```python
from build123d import *

# Parameters (mm, degrees)
F0_R     = 10
F1_DEPTH = 2


with BuildPart() as f1:
    # F0 (on Front) → F1 (new body)
    with BuildSketch(Plane.XZ):
        with BuildLine():
            ThreePointArc((-62.534281, -2.119643), (-35.69599, 2.957285), (-15.866047, -15.826814))
            Line((-15.866047, -15.826814), (10.849682, -15.826814))
            Line((10.849682, -15.826814), (10.849682, 24.173186))
            ThreePointArc((10.849682, 24.173186), (-10.750328, 10.703225), (-13.3423, 36.026771))
            Line((-13.3423, 36.026771), (-62.534281, -2.119643))
        make_face()
        with BuildLine():
            ThreePointArc((10.849682, 24.173186), (2.449692, 37.643148), (-13.3423, 36.026771))
            ThreePointArc((-13.3423, 36.026771), (-10.750328, 10.703225), (10.849682, 24.173186))
        make_face()
        with Locations((-4.150318, 24.173186)):
            Circle(F0_R, mode=Mode.SUBTRACT)
        with BuildLine():
            Line((-44.150318, -15.826814), (-15.866047, -15.826814))
            ThreePointArc((-15.866047, -15.826814), (-35.69599, 2.957285), (-62.534281, -2.119643))
            ThreePointArc((-62.534281, -2.119643), (-61.408556, -50.365624), (-15.62346, -35.1122))
            Line((-15.62346, -35.1122), (-43.898783, -35.82365))
            ThreePointArc((-43.898783, -35.82365), (-54.149527, -25.952591), (-44.150318, -15.826814))
        make_face()
    extrude(amount=F1_DEPTH)


solid = f1.part
```
Geometry check sheet. Reference: the model listing, model coordinates, mm. Give positions to 0.01 mm unless a question says otherwise; leave off trailing zeros. Order: outer loops, then holes, each group sorted by start corner. A loop starts at its lowest first (then second) coordinate and runs counter-clockwise, first axis right, second up. Notation, with made-up numbers: (83, 29.5) - (100, 29.5) arc R21 ccw to (100, 62.5) - close; hole circle Ø4 at (-22, 26). An arc over 180 degrees is marked (long way). Answer in a Markdown table with one row per item. Add a question column.
Q1. Material ranges on probe 1 along Z at (x, y) = (-4, -0.1); probe 2 along X at (y, z) = (-0.5, 26); probe 3 along X at (y, z) = (-0.5, 20.5), recorded low to high. Write a range as from..to.
Q2. Cross-section at A-A, the plane x = -39. Enter the section's corners in (y, z).
Q3. Cross-section at B-B, the plane y = -1.1. Enter the section's corners in (x, z).
Q4. Cross-section at D-D, the plane z = -44. Enter the section's corners in (x, y), then the cut area to 3 significant figures.
Q5. Cross-section at C-C, the plane x = -8. Enter the section's corners in (y, z), then the cut area to 3 significant figures.
Q6. Gauge pin test, flat ends, axial feed: pin 1 (1 mm diameter, centred on x = -48.5, y = -0.5, fed in from +Z); pin 2 (1 mm diameter, centred on x = -37.5, y = -0.5, fed in from +Z); pin 3 (10 mm diameter, centred on x = -42, z = -21, fed in from -Y). Record the tip position at first contact, or that the pin passes through.
Q7. Mould release check, pull along Z, two halves, no side actions. Record for faces 1 (the cylindrical face through (2.66, -0.99, 37.54)), 2 (the cylindrical face through (5.087, -0.986, 20.343)), 3 (the flat face through (-17, -1, -15.827)), 4 (the cylindrical face through (-62.04, -0.99, -49.91)): pulls with the +Z half, pulls with the -Z half, needs draft (parallel to the pull), parting line crosses it, or undercut.
Check values:
| question | item | result |
|---|---|---|
| 1 | probe 1 | z = -15.83..14.17, 34.17..39.17 |
| 1 | probe 2 | x = -26.27..-13.98, 5.68..10.74 |
| 1 | probe 3 | x = -33.36..-13.45, 5.15..10.85 |
| 2 | outline | (-2, -55.38) - (0, -55.38) - (0, -35.7) - (-2, -35.7) - close; (-2, -15.83) - (0, -15.83) - (0, 16.13) - (-2, 16.13) - close |
| 3 | outline | (-62.53, -2.12) arc R30 ccw (long way) to (-15.62, -35.11) - (-43.9, -35.82) arc R10 cw (long way) to (-44.15, -15.83) - (10.85, -15.83) - (10.85, 24.17) arc R15 ccw to (-13.34, 36.03) - close; hole circle Ø20 at (-4.15, 24.17) |
| 4 | outline | (-68.02, -2) - (-20.28, -2) - (-20.28, 0) - (-68.02, 0) - close |
| 4 | area | 95.5 mm^2 |
| 5 | outline | (-2, -15.83) - (0, -15.83) - (0, 14.94) - (-2, 14.94) - close; (-2, 33.4) - (0, 33.4) - (0, 38.67) - (-2, 38.67) - close |
| 5 | area | 72.1 mm^2 |
| 6 | pin 1 | stops at z = 9.15 |
| 6 | pin 2 | stops at z = 17.68 |
| 6 | pin 3 | passes through |
| 7 | face 1 | pulls with the +Z half |
| 7 | face 2 | undercut |
| 7 | face 3 | undercut |
| 7 | face 4 | parting line crosses it |
